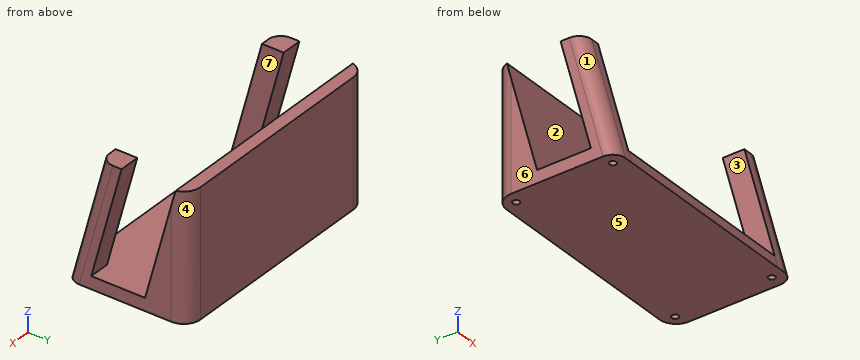
```python
from build123d import *

# Parameters (mm, degrees)
PAD_DEPTH    = 5
PAD001_DEPTH = 51.5
PAD002_DEPTH = 5
FILLET_R     = 3
FILLET001_R  = 4
SKETCH003_R  = 0.8
HOLE_DEPTH   = 3
HOLE_TIPS_R  = 0.8


with BuildPart() as part:
    # Sketch → Pad (new body)
    with BuildSketch(Plane.YZ):
        Polygon((0, 0), (8.038476, 30), (13.214857, 30), (5.980228, 3), (18.817653, 3), (26.052281, 30), (29.052281, 30), (29.052281, 0), align=None)
    extrude(amount=PAD_DEPTH)

    # Sketch001 → Pad001 (join)
    with BuildSketch(Plane.YZ):
        Polygon((0, 0), (29.052281, 0), (29.052281, 30), (26.052281, 30), (18.817653, 3), (0.803848, 3), align=None)
    extrude(amount=PAD001_DEPTH)

    # Sketch002 (on Face14 of Pad001) → Pad002 (join)
    with BuildSketch(Plane.YZ.offset(51.5)):
        Polygon((0, 0), (8.038476, 30), (13.214857, 30), (5.980228, 3), (18.817653, 3), (26.052281, 30), (29.052281, 30), (29.052281, 0), align=None)
    extrude(amount=PAD002_DEPTH)

    # Fillet
    fillet_edges = [part.edges().sort_by_distance(p)[0] for p in [
        (0, 4.421162, 16.5),
        (0, 0.401924, 1.5),
        (56.5, 4.019238, 15),
    ]]
    fillet(fillet_edges, radius=FILLET_R)

    # Fillet001
    fillet001_edges = [part.edges().sort_by_distance(p)[0] for p in [
        (0, 29.052281, 15),
        (56.5, 29.052281, 15),
    ]]
    fillet(fillet001_edges, radius=FILLET001_R)

    # Sketch003 (on Face13 of Pad002) → Hole (cut)
    with BuildSketch(Plane.YX):
        with Locations((3, 53.5)):
            Circle(SKETCH003_R)
        with Locations((26.052281, 53.5)):
            Circle(SKETCH003_R)
        with Locations((3, 3)):
            Circle(SKETCH003_R)
        with Locations((26.052281, 3)):
            Circle(SKETCH003_R)
    extrude(amount=-HOLE_DEPTH, mode=Mode.SUBTRACT)

    # Hole tips → Hole tip 1 section 0
    with BuildSketch(Plane.YX.offset(-3), mode=Mode.PRIVATE) as hole_tip_1_s0:
        with Locations((3, 53.5)):
            Circle(HOLE_TIPS_R)
    loft([hole_tip_1_s0.sketch, Vertex(53.5, 3, 3.480688)], mode=Mode.SUBTRACT)

    # Hole tips → Hole tip 2 section 0
    with BuildSketch(Plane.YX.offset(-3), mode=Mode.PRIVATE) as hole_tip_2_s0:
        with Locations((26.052281, 53.5)):
            Circle(HOLE_TIPS_R)
    loft([hole_tip_2_s0.sketch, Vertex(53.5, 26.052281, 3.480688)], mode=Mode.SUBTRACT)

    # Hole tips → Hole tip 3 section 0
    with BuildSketch(Plane.YX.offset(-3), mode=Mode.PRIVATE) as hole_tip_3_s0:
        with Locations((3, 3)):
            Circle(HOLE_TIPS_R)
    loft([hole_tip_3_s0.sketch, Vertex(3, 3, 3.480688)], mode=Mode.SUBTRACT)

    # Hole tips → Hole tip 4 section 0
    with BuildSketch(Plane.YX.offset(-3), mode=Mode.PRIVATE) as hole_tip_4_s0:
        with Locations((26.052281, 3)):
            Circle(HOLE_TIPS_R)
    loft([hole_tip_4_s0.sketch, Vertex(3, 26.052281, 3.480688)], mode=Mode.SUBTRACT)


solid = part.part
```
Read the model definition and answer for the solid it produces. Units are mm, in the model's axes. Face numbers are marked on the shaded views. A direction names the side the tool comes from. Coordinates: 2 decimals unless noted, no trailing zeros. Write each loop counter-clockwise with the first axis right and the second up, starting at its lowest first coordinate (ties: lowest second). Pieces come first, ordered by that corner, then holes. Notation, with made-up numbers: (87, -1) - (120, -1) arc R34 ccw to (120, 34) - close; hole circle Ø11 at (48.25, -20). An arc over 180 degrees is marked (long way). Answer as a JSON object with one key per item and string values. Group by question number.
1. Consider L1, parallel to X at y = 9.5, z = 23; L2, parallel to Y at x = 53.5, z = 2.35; L3, parallel to Z at x = 43.5, y = 2.5. Determine where each line is inside the solid, lowest interval first. Write a range as [from, to].
2. The mould has two halves that part along X. Classify the marked faces 4, 5, 6 and 7: +X half, -X half, draft (parallel to the pull), parting line (faces both ways), or undercut.
3. A cutting plane is placed at C-C (z = 5.5). Give the number of separate pieces and of enclosed holes in the cut face, plus the area to 3 significant figures.
4. Which of the six approach directions +Z, -Z, +X, -X, +Y, -Y give full straight-line access (tool end or side, diameter ignored) to the marked faces 1, 2 and 3?
5. Each of these flat-tipped pins is pushed along its axis until it touches: P1, Ø1, axis at x = 19, y = 9.5, coming from the -Z side; P2, Ø1, axis at x = 33.5, z = 25.5, coming from the -Y side; P3, Ø5.5, axis at x = 32.5, y = 11.5, coming from the +Z side; P4, Ø1.3, axis at x = 53.5, y = 26.05, coming from the -Z side. Where does it stop, or does it pass through?
6. A cutting plane is placed at B-B (y = 14.75). Determine the outline of the cut face in (x, z), plus the area to 4 significant figures.
7. A cutting plane is placed at A-A (x = 45). Determine the outline of the cut face in (y, z), plus the area to 3 significant figures.
Worked out:
{
 "1": {"L1": "x = [0, 5], [51.5, 56.5]", "L2": "y = [0.63, 2.2], [3.8, 25.25], [26.85, 28.93]", "L3": "z = [0, 3]"},
 "2": {"face 4": "+X half", "face 5": "draft", "face 6": "-X half", "face 7": "undercut"},
 "3": {"separate pieces": "3", "enclosed holes": "0", "area": "581 mm²"},
 "4": {"face 1": "+Z, -X, -Y", "face 2": "+Z, +X, -X", "face 3": "+Z, -Y"},
 "5": {"P1": "stops at z = 0", "P2": "stops at y = 24.71", "P3": "stops at z = 3", "P4": "stops at z = 3.09"},
 "6": {"outline": "(0, 0) - (56.5, 0) - (56.5, 3) - (0, 3) - close", "area": "169.5 mm²"},
 "7": {"outline": "(0, 0) - (29.05, 0) - (29.05, 30) - (26.05, 30) - (18.82, 3) - (0.8, 3) - close", "area": "265 mm²"}
}
